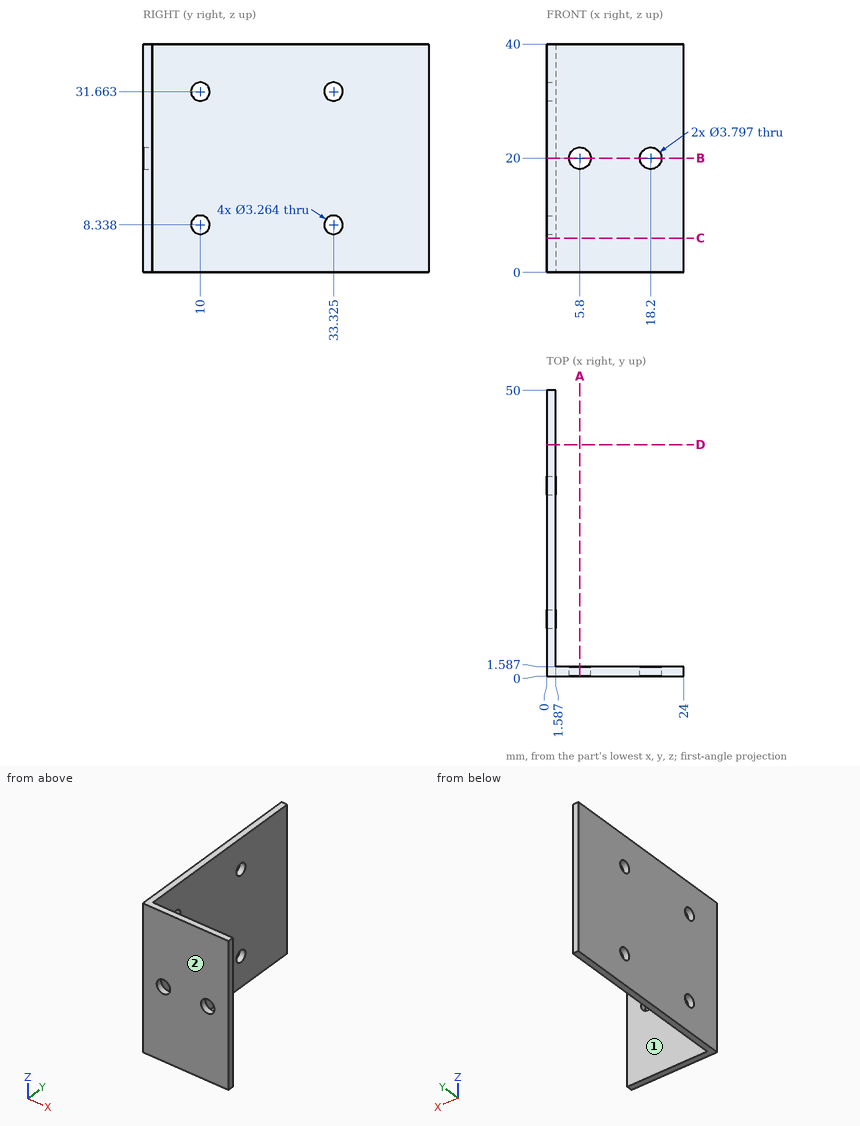
Geometry: see drawing. Coordinates: mm, zero at the bounding-box minimum. A direction names the side the tool comes from. Give positions to 0.01 mm unless a question says otherwise; leave off trailing zeros. Loops run counter-clockwise (first coordinate to the right, second up) from the corner with the lowest first, then second, coordinate; pieces in that order, holes last. Notation, with made-up numbers: (38.25, 5.25) - (86.25, 5.25) arc R21 ccw to (86.25, 34.25) - close; hole circle Ø8 at (-18.5, 2). An arc over 180 degrees is marked (long way). Use CSV: the item, a comma, the result in double quotes. Start each with the question number.
Item 1: Line query: line 1 (Z direction, x = 5.8, y = 0.85); line 2 (Y direction, x = 2.5, z = 19). Output: solid intervals per line, ascending.
Item 2: Reachability of the marked faces 1 and 2 from +Z, -Z, +X, -X, +Y, -Y: full face, straight path, thin tool, end or side. Return the list, or none.
Item 3: Section A-A on x = 5.8. Return loops of the section in (y, z).
Item 4: Section B-B on z = 20. Return loops of the section in (x, y), then the cut area to 3 significant figures.
Item 5: Section C-C on z = 6. Return loops of the section in (x, y), then the cut area to 3 significant figures.
Item 6: Section D-D on y = 40.5. Return loops of the section in (x, z).
Item 7: Contact query for flat-ended pins moving along their axis: P1, Ø6.5, axis at x = 8, z = 12, coming from the +Y side; P2, Ø6, axis at y = 38.5, z = 6.5, coming from the +X side. Output: stop coordinate, or through.
Ans:
1,line 1,"z = 0 to 18.1, 21.9 to 40"
1,line 2,"y = 0 to 1.59"
2,face 1,"+Z, -Z, +X, +Y"
2,face 2,"+Z, -Z, +X, -X, -Y"
3,outline,"(0, 0) - (1.59, 0) - (1.59, 18.1) - (0, 18.1) - close; (0, 21.9) - (1.59, 21.9) - (1.59, 40) - (0, 40) - close"
4,outline,"(0, 0) - (3.9, 0) - (3.9, 1.59) - (1.59, 1.59) - (1.59, 50) - (0, 50) - close; (7.7, 0) - (16.3, 0) - (16.3, 1.59) - (7.7, 1.59) - close; (20.1, 0) - (24, 0) - (24, 1.59) - (20.1, 1.59) - close"
4,area,"103 mm2"
5,outline,"(0, 0) - (24, 0) - (24, 1.59) - (1.59, 1.59) - (1.59, 50) - (0, 50) - close"
5,area,"115 mm2"
6,outline,"(0, 0) - (1.59, 0) - (1.59, 40) - (0, 40) - close"
7,P1,"stops at y = 1.59"
7,P2,"stops at x = 1.59"
